Part model, mm, in its own coordinate system. A direction names the side the tool comes from. Coordinates: 2 decimals unless noted, no trailing zeros. Loops run counter-clockwise (first coordinate to the right, second up) from the corner with the lowest first, then second, coordinate; pieces in that order, holes last. Notation, with made-up numbers: M -33.5,-23 L -18.5,-23 A14 cw -18.5,-18 Z; hole C -12.5,45.25 d5. An arc over 180 degrees is marked long. Use a Markdown table: item, result. Add a question column.
1) Pull direction X, two halves, no side cores. Call faces 1 (the flat face through (-39, -7, -8)), 2 (the flat face through (3, -14, -19)), 3 (the flat face through (36, -7, -11)): released by +X, released by -X, zero draft, split by the parting line, or undercut.
2) Wall check: probe 1 along X at (y, z) = (-7, -18.2); probe 2 along X at (y, z) = (-7, -19.1); probe 3 along X at (y, z) = (-9.5, -10.75). Give the ranges that are in metal, low to high. Write a range as from..to.
3) Band-saw the part on A-A (y = -7). State how many separate pieces and enclosed holes the cut face has, plus the area to 3 significant figures.
4) Band-saw the part on C-C (x = -32). List the corners of the cut face in (y, z), plus the area to 3 significant figures.
5) Tool access for faces 4 (the cylindrical face through (-29, -7, -19)), 5 (the flat face through (32, -7, -17)), 6 (the flat face through (-33.3, -7, -1)): list every direction of +Z, -Z, +X, -X, +Y, -Y with a clear straight run to the whole face (end or side of a thin tool).
6) Pin check, flat tips, straight feed: pin 1 Ø0.9 at (x, z) = (-31.5, -1) entering from -Y; pin 2 Ø3 at (x, y) = (-20, -8.5) entering from +Z. Stop position of each tip, or through.
7) Band-saw the part on D-D (z = -13.5). List the corners of the cut face in (x, y).
8) Band-saw the part on B-B (x = 30). List the corners of the cut face in (y, z).
from build123d import *

# Parameters (mm, degrees)
PAD_DEPTH    = 14
SKETCH001_R  = 1
POCKET_DEPTH = 5
SKETCH002_W  = 5
SKETCH002_H  = 3
PAD001_DEPTH = 1


with BuildPart() as part:
    # Sketch → Pad (new body)
    with BuildSketch(Plane.XZ):
        Polygon((-33.3, 0), (-33.3, -1.8), (-29, -1.8), (-29, -4.8), (-36, -4.8), (-36, -17), (-25.5, -17), (-25.5, -18.5), (25.5, -18.5), (25.5, -17), (36, -17), (36, -4.8), (29, -4.8), (29, -1.8), (33.3, -1.8), (33.3, 0), (29, 0), (29, 4.5), (39, 4.5), (39, -20), (-39, -20), (-39, 4.5), (-29, 4.5), (-29, 0), align=None)
    extrude(amount=PAD_DEPTH)

    # Sketch001 (on Face21 of Pad) → Pocket (cut)
    with BuildSketch(Plane(origin=(0, 0, -20), x_dir=(1, 0, 0), z_dir=(0, 0, -1))):
        with Locations((-30, 7)):
            Circle(SKETCH001_R)
        with Locations((30, 7)):
            Circle(SKETCH001_R)
    extrude(amount=-POCKET_DEPTH, mode=Mode.SUBTRACT)

    # Sketch002 (on Face4 of Pocket) → Pad001 (join)
    with BuildSketch(Plane(origin=(0, 0, 0), x_dir=(1, 0, 0), z_dir=(0, 1, 0))):
        with Locations((-31.5, 1)):
            Rectangle(SKETCH002_W, SKETCH002_H)
        with Locations((31.5, 1)):
            Rectangle(SKETCH002_W, SKETCH002_H)
    extrude(amount=-PAD001_DEPTH)


solid = part.part
Entries:
| question | item | result |
|---|---|---|
| 1 | face 1 | released by -X |
| 1 | face 2 | zero draft |
| 1 | face 3 | undercut |
| 2 | probe 1 | -39..-31, -29..-25.5, 25.5..29, 31..39 |
| 2 | probe 2 | -39..-31, -29..29, 31..39 |
| 2 | probe 3 | -39..-36, 36..39 |
| 3 | separate pieces | 3 |
| 3 | enclosed holes | 0 |
| 3 | area | 389 mm2 |
| 4 | outline | M -14,-20 L 0,-20 L 0,-17 L -14,-17 Z; M -14,-4.8 L 0,-4.8 L 0,4.5 L -14,4.5 L -14,0 L -1,0 L -1,-1.8 L -14,-1.8 Z |
| 4 | area | 149 mm2 |
| 5 | face 4 | -Z |
| 5 | face 5 | +Y, -Y |
| 5 | face 6 | -Y |
| 6 | pin 1 | y = -1 |
| 6 | pin 2 | z = -18.5 |
| 7 | outline | M -39,-14 L -36,-14 L -36,0 L -39,0 Z; M 36,-14 L 39,-14 L 39,0 L 36,0 Z |
| 8 | outline | M -14,-20 L -8,-20 L -8,-17 L -14,-17 Z; M -14,-4.8 L 0,-4.8 L 0,4.5 L -14,4.5 L -14,0 L -1,0 L -1,-1.8 L -14,-1.8 Z; M -6,-20 L 0,-20 L 0,-17 L -6,-17 Z |
